For this review, take the finished solid that the model builds, in its own axes (mm). A direction names the side the tool comes from. Round coordinates to 2 decimals unless told otherwise and drop trailing zeros. Write each loop counter-clockwise with the first axis right and the second up, starting at its lowest first coordinate (ties: lowest second). Pieces come first, ordered by that corner, then holes. Notation, with made-up numbers: (-29.75, 18) -> (5.25, 18) arc R26 cw to (5.25, 52) -> close; hole circle Ø2 at (28.5, 60.5). An arc over 180 degrees is marked (long way). Answer in a Markdown table with one row per item.
from build123d import *

# Parameters (mm, degrees)
SKETCH1_R           = 72.5
BOSS_EXTRUDE1_DEPTH = 25
SKETCH1_4_R         = 72.5
SKETCH1_4_R_2       = 14.5
BOSS_EXTRUDE2_DEPTH = 1
SKETCH1_5_R         = 72.5
SKETCH1_5_R_2       = 18.375
BOSS_EXTRUDE3_DEPTH = 7
SKETCH1_8_R         = 72.5
SKETCH1_8_R_2       = 49.75
BOSS_EXTRUDE5_DEPTH = 9
SKETCH1_10_R        = 72.5
SKETCH1_10_R_2      = 53.375
BOSS_EXTRUDE6_DEPTH = 15
SKETCH1_11_R        = 1.65
CUT_EXTRUDE1_DEPTH  = 26
SKETCH1_12_R        = 3
CUT_EXTRUDE2_DEPTH  = 8
SKETCH1_15_R        = 1.65
CUT_EXTRUDE3_DEPTH  = 20
CUT_EXTRUDE4_START  = 7
SKETCH1_16_R        = 3
CUT_EXTRUDE4_DEPTH  = 3.1


with BuildPart() as part:
    # Sketch1 → Boss-Extrude1 (new body)
    with BuildSketch(Plane(origin=(0, 0, 0), x_dir=(1, 0, 0), z_dir=(0, 1, 0))):
        with Locations((-0.792166463, -0.608066556)):
            Circle(SKETCH1_R)
        with BuildLine():
            ThreePointArc((-63.593753764, -5.604128245), (-58.792166463, -0.608066556), (-63.593753764, 4.387995133))
            ThreePointArc((-63.593753764, 4.387995133), (-63.150917301, 8.357768256), (-62.457401444, 12.291499122))
            ThreePointArc((-62.457401444, 12.291499122), (-56.442758932, 15.732421741), (-59.642294977, 21.878871295))
            ThreePointArc((-59.642294977, 21.878871295), (-58.09898217, 25.563079263), (-56.325298523, 29.142080394))
            ThreePointArc((-56.325298523, 29.142080394), (-49.584871367, 30.749100857), (-50.923148772, 37.547989487))
            ThreePointArc((-50.923148772, 37.547989487), (-48.404389647, 40.648159683), (-45.694231511, 43.582481692))
            ThreePointArc((-45.694231511, 43.582481692), (-38.774089031, 43.225408757), (-38.142688521, 50.125930941))
            ThreePointArc((-38.142688521, 50.125930941), (-34.852537962, 52.390906013), (-31.425466231, 54.442827581))
            ThreePointArc((-31.425466231, 54.442827581), (-24.886237217, 52.150589175), (-22.336311105, 58.593705644))
            ThreePointArc((-22.336311105, 58.593705644), (-18.541317544, 59.839990782), (-14.674973188, 60.843277428))
            ThreePointArc((-14.674973188, 60.843277428), (-9.046427083, 56.801577073), (-4.784555218, 62.265304851))
            ThreePointArc((-4.784555218, 62.265304851), (-0.792166463, 62.391933444), (3.200222293, 62.265304851))
            ThreePointArc((3.200222293, 62.265304851), (7.462094157, 56.801577073), (13.090640262, 60.843277428))
            ThreePointArc((13.090640262, 60.843277428), (16.956984618, 59.839990782), (20.75197818, 58.593705644))
            ThreePointArc((20.75197818, 58.593705644), (23.301904291, 52.150589175), (29.841133306, 54.442827581))
            ThreePointArc((29.841133306, 54.442827581), (33.268205037, 52.390906013), (36.558355596, 50.125930941))
            ThreePointArc((36.558355596, 50.125930941), (37.189756106, 43.225408757), (44.109898586, 43.582481692))
            ThreePointArc((44.109898586, 43.582481692), (46.820056722, 40.648159683), (49.338815847, 37.547989487))
            ThreePointArc((49.338815847, 37.547989487), (48.000538442, 30.749100857), (54.740965598, 29.142080394))
            ThreePointArc((54.740965598, 29.142080394), (56.514649245, 25.563079263), (58.057962051, 21.878871295))
            ThreePointArc((58.057962051, 21.878871295), (54.858426007, 15.732421741), (60.873068519, 12.291499122))
            ThreePointArc((60.873068519, 12.291499122), (61.566584376, 8.357768256), (62.009420839, 4.387995133))
            ThreePointArc((62.009420839, 4.387995133), (57.207833537, -0.608066556), (62.009420839, -5.604128245))
            ThreePointArc((62.009420839, -5.604128245), (61.566584376, -9.573901367), (60.873068519, -13.507632233))
            ThreePointArc((60.873068519, -13.507632233), (54.858426007, -16.948554852), (58.057962051, -23.095004406))
            ThreePointArc((58.057962051, -23.095004406), (56.514649245, -26.779212375), (54.740965598, -30.358213506))
            ThreePointArc((54.740965598, -30.358213506), (48.000538442, -31.965233968), (49.338815847, -38.764122598))
            ThreePointArc((49.338815847, -38.764122598), (46.820056722, -41.864292794), (44.109898586, -44.798614803))
            ThreePointArc((44.109898586, -44.798614803), (37.189756106, -44.441541868), (36.558355596, -51.342064052))
            ThreePointArc((36.558355596, -51.342064052), (33.268205037, -53.607039124), (29.841133306, -55.658960693))
            ThreePointArc((29.841133306, -55.658960693), (23.301904291, -53.366722286), (20.75197818, -59.809838756))
            ThreePointArc((20.75197818, -59.809838756), (16.956984618, -61.056123893), (13.090640262, -62.05941054))
            ThreePointArc((13.090640262, -62.05941054), (7.462094157, -58.017710185), (3.200222293, -63.481437962))
            ThreePointArc((3.200222293, -63.481437962), (-0.792166463, -63.608066556), (-4.784555218, -63.481437962))
            ThreePointArc((-4.784555218, -63.481437962), (-9.046427083, -58.017710185), (-14.674973188, -62.05941054))
            ThreePointArc((-14.674973188, -62.05941054), (-18.541317544, -61.056123893), (-22.336311105, -59.809838756))
            ThreePointArc((-22.336311105, -59.809838756), (-24.886237217, -53.366722286), (-31.425466231, -55.658960693))
            ThreePointArc((-31.425466231, -55.658960693), (-34.852537962, -53.607039124), (-38.142688521, -51.342064052))
            ThreePointArc((-38.142688521, -51.342064052), (-38.774089031, -44.441541868), (-45.694231511, -44.798614803))
            ThreePointArc((-45.694231511, -44.798614803), (-48.404389647, -41.864292794), (-50.923148772, -38.764122598))
            ThreePointArc((-50.923148772, -38.764122598), (-49.584871367, -31.965233968), (-56.325298523, -30.358213506))
            ThreePointArc((-56.325298523, -30.358213506), (-58.09898217, -26.779212375), (-59.642294977, -23.095004406))
            ThreePointArc((-59.642294977, -23.095004406), (-56.442758932, -16.948554852), (-62.457401444, -13.507632233))
            ThreePointArc((-62.457401444, -13.507632233), (-63.150917301, -9.573901367), (-63.593753764, -5.604128245))
        make_face(mode=Mode.SUBTRACT)
    extrude(amount=BOSS_EXTRUDE1_DEPTH)

    # Sketch1<4> → Boss-Extrude2 (add)
    with BuildSketch(Plane(origin=(0, 0, 0), x_dir=(1, 0, 0), z_dir=(0, 1, 0))):
        with Locations((-0.792166463, -0.608066556)):
            Circle(SKETCH1_4_R)
        with Locations((-0.792166463, -0.608066556)):
            Circle(SKETCH1_4_R_2, mode=Mode.SUBTRACT)
    extrude(amount=BOSS_EXTRUDE2_DEPTH)

    # Sketch1<5> → Boss-Extrude3 (add)
    with BuildSketch(Plane(origin=(0, 0, 0), x_dir=(1, 0, 0), z_dir=(0, 1, 0))):
        with Locations((-0.792166463, -0.608066556)):
            Circle(SKETCH1_5_R)
        with Locations((-0.792166463, -0.608066556)):
            Circle(SKETCH1_5_R_2, mode=Mode.SUBTRACT)
    extrude(amount=BOSS_EXTRUDE3_DEPTH)

    # Sketch1<8> → Boss-Extrude5 (add)
    with BuildSketch(Plane(origin=(0, 0, 0), x_dir=(1, 0, 0), z_dir=(0, 1, 0))):
        with Locations((-0.792166463, -0.608066556)):
            Circle(SKETCH1_8_R)
        with Locations((-0.792166463, -0.608066556)):
            Circle(SKETCH1_8_R_2, mode=Mode.SUBTRACT)
    extrude(amount=BOSS_EXTRUDE5_DEPTH)

    # Sketch1<10> → Boss-Extrude6 (add)
    with BuildSketch(Plane(origin=(0, 0, 0), x_dir=(1, 0, 0), z_dir=(0, 1, 0))):
        with Locations((-0.792166463, -0.608066556)):
            Circle(SKETCH1_10_R)
        with Locations((-0.792166463, -0.608066556)):
            Circle(SKETCH1_10_R_2, mode=Mode.SUBTRACT)
    extrude(amount=BOSS_EXTRUDE6_DEPTH)

    # Sketch1<11> → Cut-Extrude1 (cut, through all)
    with BuildSketch(Plane(origin=(0, 0, 0), x_dir=(1, 0, 0), z_dir=(0, 1, 0))):
        with Locations((-68.730033322, -0.608066556)):
            Circle(SKETCH1_11_R)
        with Locations((-34.761099892, 58.227852024)):
            Circle(SKETCH1_11_R)
        with Locations((33.176766967, 58.227852024)):
            Circle(SKETCH1_11_R)
        with Locations((67.145700397, -0.608066556)):
            Circle(SKETCH1_11_R)
        with Locations((33.176766967, -59.443985135)):
            Circle(SKETCH1_11_R)
        with Locations((-34.761099892, -59.443985135)):
            Circle(SKETCH1_11_R)
    extrude(amount=CUT_EXTRUDE1_DEPTH, mode=Mode.SUBTRACT)

    # Sketch1<12> → Cut-Extrude2 (cut)
    with BuildSketch(Plane(origin=(0, 0, 0), x_dir=(1, 0, 0), z_dir=(0, 1, 0))):
        with Locations((-68.730033322, -0.608066556)):
            Circle(SKETCH1_12_R)
        with Locations((-34.761099892, 58.227852024)):
            Circle(SKETCH1_12_R)
        with Locations((33.176766967, 58.227852024)):
            Circle(SKETCH1_12_R)
        with Locations((67.145700397, -0.608066556)):
            Circle(SKETCH1_12_R)
        with Locations((33.176766967, -59.443985135)):
            Circle(SKETCH1_12_R)
        with Locations((-34.761099892, -59.443985135)):
            Circle(SKETCH1_12_R)
    extrude(amount=CUT_EXTRUDE2_DEPTH, mode=Mode.SUBTRACT)

    # Sketch1<15> → Cut-Extrude3 (cut)
    with BuildSketch(Plane(origin=(0, 0, 0), x_dir=(1, 0, 0), z_dir=(0, 1, 0))):
        with Locations((-24.792166462, 23.391933444)):
            Circle(SKETCH1_15_R)
        with Locations((23.207833537, 23.391933444)):
            Circle(SKETCH1_15_R)
        with Locations((23.207833537, -24.608066556)):
            Circle(SKETCH1_15_R)
        with Locations((-24.792166463, -24.608066555)):
            Circle(SKETCH1_15_R)
    extrude(amount=CUT_EXTRUDE3_DEPTH, mode=Mode.SUBTRACT)

    # Sketch1<16> → Cut-Extrude4 (cut)
    with BuildSketch(Plane(origin=(0, 0, 0), x_dir=(1, 0, 0), z_dir=(0, 1, 0)).offset(CUT_EXTRUDE4_START)):
        with Locations((-24.792166462, 23.391933444)):
            Circle(SKETCH1_16_R)
        with Locations((23.207833537, 23.391933444)):
            Circle(SKETCH1_16_R)
        with Locations((23.207833537, -24.608066556)):
            Circle(SKETCH1_16_R)
        with Locations((-24.792166463, -24.608066555)):
            Circle(SKETCH1_16_R)
    extrude(amount=-CUT_EXTRUDE4_DEPTH, mode=Mode.SUBTRACT)


solid = part.part
1) Consider section B-B on y = 11.75. State the section outline as (x, z) points (3 decimals).
Solved:
| item | result |
|---|---|
| outline | circle Ø145 at (-0.792, 0.608); hole circle Ø3.3 at (-68.73, 0.608); hole circle Ø106.75 at (-0.792, 0.608); hole circle Ø3.3 at (-34.761, -58.228); hole circle Ø3.3 at (-34.761, 59.444); hole circle Ø3.3 at (33.177, -58.228); hole circle Ø3.3 at (33.177, 59.444); hole circle Ø3.3 at (67.146, 0.608) |
2) Clearance check with flat-ended pins moving along their axes: pin 1 Ø8 at (x, y) = (21.5, 20) entering from +Z; pin 2 Ø8 at (x, z) = (-19.5, 51) entering from +Y; pin 3 Ø10 at (x, y) = (-47, 4) entering from -Z; pin 4 Ø2 at (x, z) = (-24.79, -23.39) entering from -Y. State where each tip first meets the part, or that it passes through.
Solved:
| item | result |
|---|---|
| pin 1 | z = 70.76 |
| pin 2 | y = 15 |
| pin 3 | z = -59.04 |
| pin 4 | through |
3) For faces 1 (the flat face through (-45, 9, -23)), 2 (the cylindrical face through (22.993, 1.923, 22.972)), 3 (the cylindrical face through (64.15, 3.94, 0.48)), list the 3-axis set-ups (+Z, -Z, +X, -X, +Y, -Y) from which the entire face can be reached by the end or side of a thin tool; tool diameter is ignored.
Solved:
| item | result |
|---|---|
| face 1 | +Y |
| face 2 | +Y, -Y |
| face 3 | -Y |
4) For line 1 (Z direction, x = -33.5, y = 18.5); line 2 (X direction, y = 17.25, z = 1); line 3 (Z direction, x = -38, y = 17.5), list the stretches that pass through material, from the lowest coordinate up. Write a range as [from, to].
Solved:
| item | result |
|---|---|
| line 1 | [-64.09, -59.29], [-57.16, -53.24], [54.45, 58.38], [60.51, 65.31] |
| line 2 | [-73.29, -70.33], [-67.13, -58.81], [57.22, 65.54], [68.75, 71.71] |
| line 3 | [-61.62, -50.23], [-49.94, -44.07], [45.29, 51.15], [51.45, 62.83] |
5) Mouldability with a two-part tool opening along Z and no side actions: class faces 4 (the cylindrical face through (-16.509, 12.325, 71.384)), 5 (the cylindrical face through (17.01, 19.93, 61.04)), 6 (the cylindrical face through (-58.793, 19.93, 0.715)) as pulls with the +Z half, pulls with the -Z half, needs draft (parallel to the pull), parting line crosses it, or undercut.
Solved:
| item | result |
|---|---|
| face 4 | parting line crosses it |
| face 5 | undercut |
| face 6 | undercut |
6) Consider section A-A on x = -0.5. State the section outline as (y, z) points, then the cut area to 3 significant figures.
Solved:
| item | result |
|---|---|
| outline | (0, -71.89) -> (25, -71.89) -> (25, -62.39) -> (15, -62.39) -> (15, -52.77) -> (9, -52.77) -> (9, -49.14) -> (7, -49.14) -> (7, -17.76) -> (1, -17.76) -> (1, -13.89) -> (0, -13.89) -> close; (0, 15.11) -> (1, 15.11) -> (1, 18.98) -> (7, 18.98) -> (7, 50.36) -> (9, 50.36) -> (9, 53.98) -> (15, 53.98) -> (15, 63.61) -> (25, 63.61) -> (25, 73.11) -> (0, 73.11) -> close |
| area | 1,280 mm² |
